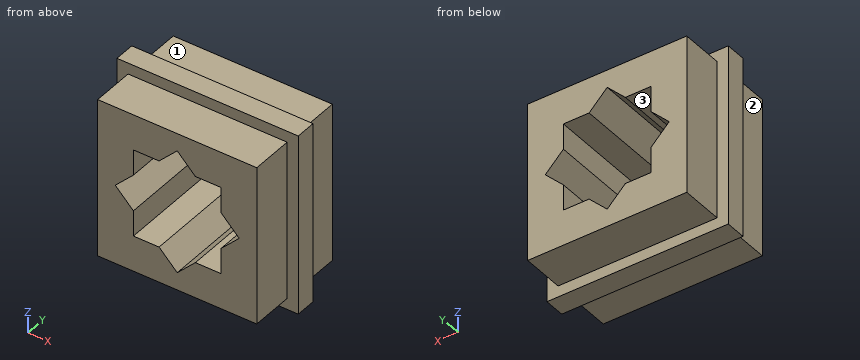
```python
from build123d import *

# Parameters (mm, degrees)
SKETCH1_W           = 25.4
SKETCH1_H           = 25.4
BOSS_EXTRUDE1_DEPTH = 8.45
SKETCH2_W           = 28.956
SKETCH2_H           = 28.956
BOSS_EXTRUDE2_DEPTH = 1.651
CUT_EXTRUDE1_DEPTH  = 17.9
CIRPATTERN1_COUNT   = 2
CIRPATTERN1_ANGLE   = 45
SKETCH4_W           = 14
SKETCH4_H           = 14
CUT_EXTRUDE2_DEPTH  = 17.9


with BuildPart() as part:
    # Sketch1 → Boss-Extrude1 (new body, symmetric)
    with BuildSketch(Plane(origin=(0, 0, 0), x_dir=(1, 0, 0), z_dir=(0, 1, 0))):
        Rectangle(SKETCH1_W, SKETCH1_H)
    extrude(amount=BOSS_EXTRUDE1_DEPTH, both=True)

    # Sketch2 → Boss-Extrude2 (add, symmetric)
    with BuildSketch(Plane(origin=(0, 0, 0), x_dir=(1, 0, 0), z_dir=(0, 1, 0))):
        Rectangle(SKETCH2_W, SKETCH2_H)
    extrude(amount=BOSS_EXTRUDE2_DEPTH, both=True)

    # Sketch3 → Cut-Extrude1 (cut, through all)
    with BuildSketch(Plane(origin=(0, 8.45, 0), x_dir=(1, 0, 0), z_dir=(0, 1, 0))):
        Polygon((-5.727922061, 7), (-7, 5.727922061), (-7, -5.727922061), (-5.727922061, -7), (5.727922061, -7), (7, -5.727922061), (7, 5.727922061), (5.727922061, 7), align=None)
    cut_extrude1 = extrude(amount=-CUT_EXTRUDE1_DEPTH, mode=Mode.SUBTRACT)

    # CirPattern1: Cut-Extrude1 ×2 about axis
    cirpattern1_axis = Axis((0, 0, 0), (0, -1, 0))
    for i in range(1, CIRPATTERN1_COUNT):
        add(cut_extrude1.rotate(cirpattern1_axis, i * CIRPATTERN1_ANGLE / (CIRPATTERN1_COUNT - 1)), mode=Mode.SUBTRACT)

    # Sketch4 → Cut-Extrude2 (cut, through all)
    with BuildSketch(Plane(origin=(0, 8.45, 0), x_dir=(1, 0, 0), z_dir=(0, 1, 0))):
        Rectangle(SKETCH4_W, SKETCH4_H)
        Polygon((0, -9.899494937), (-9.899494937, 0), (0, 9.899494937), (9.899494937, 0), align=None)
    extrude(amount=-CUT_EXTRUDE2_DEPTH, mode=Mode.SUBTRACT)


solid = part.part
```
Source: CAD feature listing. Evaluate the final solid. Frame: model axes, mm. Face numbers are marked on the shaded views. A direction names the side the tool comes from. Give positions to 0.01 mm unless a question says otherwise; leave off trailing zeros. Order: outer loops, then holes, each group sorted by start corner. A loop starts at its lowest first (then second) coordinate and runs counter-clockwise, first axis right, second up.
(1) Section query B-B (y = 5). Return the cut outline in (x, z), plus the area to 3 significant figures.
(2) Section query A-A (z = -3.5). Return the cut outline in (x, y).
(3) Contact query for flat-ended pins moving along their axis: P1, Ø2, axis at x = -6, y = -6.5, coming from the -Z side; P2, Ø6, axis at x = -4.5, y = -5, coming from the +Z side; P3, Ø2, axis at y = 6, z = -4.5, coming from the -X side; P4, Ø7.5, axis at y = 4.5, z = 1.5, coming from the +X side. Output: stop coordinate, or through.
(4) Section query C-C (x = 8.5). Return the cut outline in (y, z), plus the area to 3 significant figures.
(5) Access query for the marked faces 1, 2 and 3. Directions: +Z, -Z, +X, -X, +Y, -Y. A direction counts if a zero-diameter tool reaches every point of the face in a straight line with its end or side. Return the directions, or none.
(6) Section query D-D (z = -12). Return the cut outline in (x, y).
(7) Material intervals for line 1 along Z through (x, y) = (6, 5); line 2 along X through (y, z) = (1.25, -6), sorted ascending.
Outcome:
1. outline: (-12.7, -12.7) - (12.7, -12.7) - (12.7, 12.7) - (-12.7, 12.7) - close; hole (-9.9, 0) - (-7, -2.9) - (-7, -7) - (-2.9, -7) - (0, -9.9) - (2.9, -7) - (7, -7) - (7, -2.9) - (9.9, 0) - (7, 2.9) - (7, 7) - (2.9, 7) - (0, 9.9) - (-2.9, 7) - (-7, 7) - (-7, 2.9) - close
1. area: 416 mm2
2. outline: (-14.48, -1.65) - (-12.7, -1.65) - (-12.7, -8.45) - (-7, -8.45) - (-7, 8.45) - (-12.7, 8.45) - (-12.7, 1.65) - (-14.48, 1.65) - close; (7, -8.45) - (12.7, -8.45) - (12.7, -1.65) - (14.48, -1.65) - (14.48, 1.65) - (12.7, 1.65) - (12.7, 8.45) - (7, 8.45) - close
3. P1: stops at z = -12.7
3. P2: stops at z = 12.7
3. P3: stops at x = -12.7
3. P4: stops at x = 14.48
4. outline: (-8.45, -12.7) - (-1.65, -12.7) - (-1.65, -14.48) - (1.65, -14.48) - (1.65, -12.7) - (8.45, -12.7) - (8.45, -1.4) - (-8.45, -1.4) - close; (-8.45, 1.4) - (8.45, 1.4) - (8.45, 12.7) - (1.65, 12.7) - (1.65, 14.48) - (-1.65, 14.48) - (-1.65, 12.7) - (-8.45, 12.7) - close
4. area: 394 mm2
5. face 1: +Z, +X, -X, +Y
5. face 2: +Z, -Z, -X, -Y
5. face 3: +Y, -Y
6. outline: (-14.48, -1.65) - (-12.7, -1.65) - (-12.7, -8.45) - (12.7, -8.45) - (12.7, -1.65) - (14.48, -1.65) - (14.48, 1.65) - (12.7, 1.65) - (12.7, 8.45) - (-12.7, 8.45) - (-12.7, 1.65) - (-14.48, 1.65) - close
7. line 1: z = -12.7 to -7, 7 to 12.7
7. line 2: x = -14.48 to -7, 7 to 14.48
